```python
from build123d import *

# Parameters (mm, degrees)
F0_W     = 38.1
F0_H     = 25.4
F1_DEPTH = 12.7
F2_W     = 34.925
F2_H     = 22.225
F3_DEPTH = 1.5875
F4_R     = 0.762
F5_R     = 0.254
F6_W     = 7.1628
F6_H     = 2.032
F7_DEPTH = 25.4


with BuildPart() as f1:
    # F0 (on Top) → F1 (new body)
    with BuildSketch(Plane.XY):
        Rectangle(F0_W, F0_H)
    extrude(amount=F1_DEPTH)

    # F2 (on face) → F3 (cut)
    with BuildSketch(Plane.XY.offset(12.7)):
        Rectangle(F2_W, F2_H)
    extrude(amount=-F3_DEPTH, mode=Mode.SUBTRACT)

    # F4
    f4_edges = [f1.edges().sort_by_distance(p)[0] for p in [
        (-19.05, -12.7, 6.35),
        (-19.05, 12.7, 6.35),
        (19.05, 12.7, 6.35),
        (19.05, -12.7, 6.35),
    ]]
    fillet(f4_edges, radius=F4_R)

    # F5
    f5_edges = [f1.edges().sort_by_distance(p)[0] for p in [
        (0, 12.7, 12.7),
        (18.826815, 12.476815, 12.7),
        (-18.826815, 12.476815, 12.7),
        (19.05, 0, 12.7),
        (-19.05, 0, 12.7),
        (18.826815, -12.476815, 12.7),
        (-18.826815, -12.476815, 12.7),
        (0, -12.7, 12.7),
        (0, 11.1125, 12.7),
        (-17.4625, 0, 12.7),
        (0, -11.1125, 12.7),
        (17.4625, 0, 12.7),
    ]]
    fillet(f5_edges, radius=F5_R)

    # F6 (on Top) → F7 (cut)
    with BuildSketch(Plane.XY):
        with Locations((-10.7061, -7.62)):
            Rectangle(F6_W, F6_H)
        with Locations((-9.91108, 0)):
            Rectangle(F6_W, F6_H)
        with Locations((-8.32358, 7.62)):
            Rectangle(F6_W, F6_H)
        with Locations((10.0658737301, 3.81)):
            Rectangle(F6_W, F6_H)
        Polygon((9.198520352, -2.794), (6.4844737301, -2.794), (6.4844737301, -4.826), (8.8766831692, -4.826), align=None)
        Polygon((9.620991022, -0.126625167), (9.198520352, -2.794), (11.2558494876, -2.794), (11.6279737301, -0.4445), align=None)
        Polygon((11.2558494876, -2.794), (9.198520352, -2.794), (8.8766831692, -4.826), (10.9340123049, -4.826), align=None)
        Polygon((13.6472737301, -2.794), (11.2558494876, -2.794), (10.9340123049, -4.826), (13.6472737301, -4.826), align=None)
        Polygon((10.9340123049, -4.826), (8.8766831692, -4.826), (8.5032636406, -7.1836781144), (10.5074649439, -7.519114046), align=None)
        Polygon((5.0164880452, 0.3089470527), (6.1342154266, 7.366), (4.1272327185, 7.683874833), (3.0095053371, 0.6268218856), align=None)
        Polygon((3.7370418425, -7.7691583474), (4.8575506287, -0.6945443014), (2.8505679206, -0.3766694684), (1.7300591344, -7.4512835144), align=None)
    extrude(amount=F7_DEPTH, mode=Mode.SUBTRACT)


solid = f1.part
```
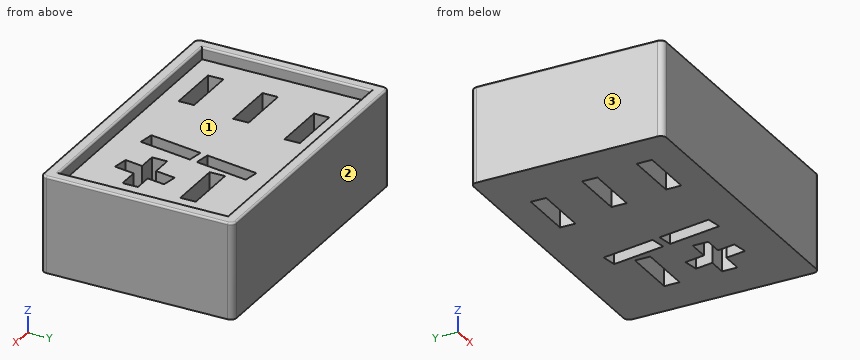
Work out the finished part from the listing and answer in its coordinate system (mm). Face numbers are marked on the shaded views. Round coordinates to 2 decimals unless told otherwise and drop trailing zeros. Write each loop counter-clockwise with the first axis right and the second up, starting at its lowest first coordinate (ties: lowest second). Pieces come first, ordered by that corner, then holes. Notation, with made-up numbers: (89.25, -29.5) - (134.25, -29.5) arc R25 ccw to (134.25, 7.5) - close; hole circle Ø2 at (12.5, 46). An arc over 180 degrees is marked (long way). Return JSON: item names as keys, results as strings. Group by question number.
Q1. The part is cut by section C-C on y = -10.5. Write down the section's boundary in (x, z).
Q2. The part is cut by section B-B on x = -9. Write down the section's boundary in (y, z).
Q3. The mould has two halves that part along X. Classify the marked faces 1, 2 and 3: released by +X, released by -X, zero draft, split by the parting line, or undercut.
Q4. The part is cut by section D-D on z = 11.5. Write down the section's boundary in (x, y), then the cut area to 3 significant figures.
Q5. The part is cut by section A-A on x = 7.5. Write down the section's boundary in (y, z), then the cut area to 3 significant figures.
Q6. Find the intervals of material crossed by L1, parallel to Y at x = -7, z = 2; L2, parallel to Y at x = -7.5, z = 9; L3, parallel to Y at x = 11, z = 2, in increasing order.
Q7. This flat-tipped pin is pushed along its axis until it touches: pin 1 Ø6 at (x, y) = (11, 1.5) entering from +Z. Where does it stop, or does it pass through?
Solved:
{
 "1": {"outline": "(-19.05, 0) - (19.05, 0) - (19.05, 12.45) arc R0.25 ccw to (18.8, 12.7) - (17.72, 12.7) arc R0.25 ccw to (17.46, 12.45) - (17.46, 11.11) - (-17.46, 11.11) - (-17.46, 12.45) arc R0.25 ccw to (-17.72, 12.7) - (-18.8, 12.7) arc R0.25 ccw to (-19.05, 12.45) - close"},
 "2": {"outline": "(-12.7, 0) - (-8.64, 0) - (-8.64, 11.11) - (-11.11, 11.11) - (-11.11, 12.45) arc R0.25 ccw to (-11.37, 12.7) - (-12.45, 12.7) arc R0.25 ccw to (-12.7, 12.45) - close; (-6.6, 0) - (-1.02, 0) - (-1.02, 11.11) - (-6.6, 11.11) - close; (1.02, 0) - (6.6, 0) - (6.6, 11.11) - (1.02, 11.11) - close; (8.64, 0) - (12.7, 0) - (12.7, 12.45) arc R0.25 ccw to (12.45, 12.7) - (11.37, 12.7) arc R0.25 ccw to (11.11, 12.45) - (11.11, 11.11) - (8.64, 11.11) - close"},
 "3": {"face 1": "undercut", "face 2": "zero draft", "face 3": "released by -X"},
 "4": {"outline": "(-19.05, -11.94) arc R0.76 ccw to (-18.29, -12.7) - (18.29, -12.7) arc R0.76 ccw to (19.05, -11.94) - (19.05, 11.94) arc R0.76 ccw to (18.29, 12.7) - (-18.29, 12.7) arc R0.76 ccw to (-19.05, 11.94) - close; hole (-17.46, -11.11) - (17.46, -11.11) - (17.46, 11.11) - (-17.46, 11.11) - close", "area": "191 mm²"},
 "5": {"outline": "(-12.7, 0) - (-4.83, 0) - (-4.83, 11.11) - (-11.11, 11.11) - (-11.11, 12.45) arc R0.25 ccw to (-11.37, 12.7) - (-12.45, 12.7) arc R0.25 ccw to (-12.7, 12.45) - close; (-2.79, 0) - (2.79, 0) - (2.79, 11.11) - (-2.79, 11.11) - close; (4.83, 0) - (12.7, 0) - (12.7, 12.45) arc R0.25 ccw to (12.45, 12.7) - (11.37, 12.7) arc R0.25 ccw to (11.11, 12.45) - (11.11, 11.11) - (4.83, 11.11) - close", "area": "242 mm²"},
 "6": {"L1": "-12.7 to -1.02, 1.02 to 6.6, 8.64 to 12.7", "L2": "-12.7 to -8.64, -6.6 to -1.02, 1.02 to 6.6, 8.64 to 12.7", "L3": "-12.7 to -4.83, -0.35 to 2.79, 4.83 to 12.7"},
 "7": {"pin 1": "z = 11.11"}
}
